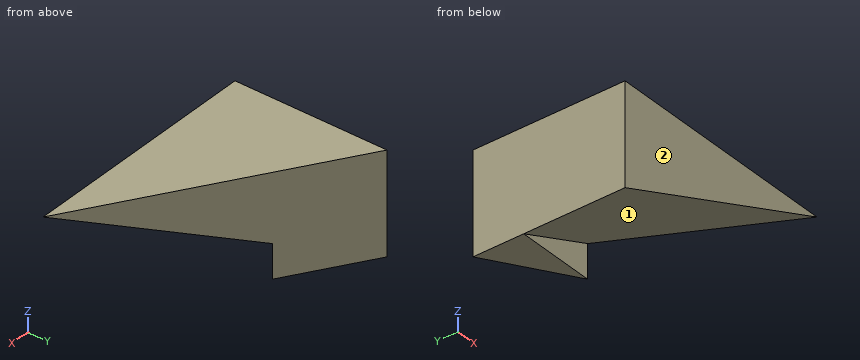
from build123d import *

# Parameters (mm, degrees)
F1_DEPTH = 25
F3_DEPTH = 25


with BuildPart() as f1:
    # F0 (on Top) → F1 (new body)
    with BuildSketch(Plane.XY):
        Polygon((-59.480719, 22.291102), (-118.588671, 59.791102), (-118.588671, 22.291102), align=None)
    extrude(amount=F1_DEPTH)

    # F2 (on face) → F3 (cut)
    with BuildSketch(Plane.XZ.offset(-22.291102)):
        Polygon((-59.480719, 25), (-118.588671, 0), (-59.480719, 0), align=None)
    extrude(amount=-F3_DEPTH, mode=Mode.SUBTRACT)


solid = f1.part
The listing builds one solid part. Answer for the finished solid, in the listing's coordinates (mm). Face numbers are marked on the shaded views. A direction names the side the tool comes from. Round coordinates to 2 decimals unless told otherwise and drop trailing zeros. Write each loop counter-clockwise with the first axis right and the second up, starting at its lowest first coordinate (ties: lowest second). Pieces come first, ordered by that corner, then holes. Notation, with made-up numbers: M -8.5,44 L 50.5,44 A17 ccw 50.5,69 Z; hole C 46.5,22 d7. An arc over 180 degrees is marked long. Write each question's results on one line, items separated by ' | '. Start each with the question number.
Item 1: Find section D-D on z = 4. Write down the section's boundary in (x, y), and give its area (3 significant figures).
Item 2: Straight lines are drawn through the part: probe 1 along X at (y, z) = (43, 1); probe 2 along Z at (x, y) = (-101.5, 41); probe 3 along Y at (x, z) = (-101, 7.25). For each, find the intervals that lie inside material, in ascending order.
Item 3: Given pin 1 Ø3 at (x, y) = (-110, 37.5) entering from -Z; pin 2 Ø4 at (x, y) = (-83, 36) entering from -Z, each flat-ended and moving along its own axis, determine where each tip first touches the part or whether it passes through.
Item 4: Find section C-C on y = 56. Write down the section's boundary in (x, z).
Item 5: Which of the six approach directions +Z, -Z, +X, -X, +Y, -Y give full straight-line access (tool end or side, diameter ignored) to the marked faces 1 and 2?
Item 6: Find section A-A on x = -104. Write down the section's boundary in (y, z), and give its area (3 significant figures).
Item 7: Find section B-B on z = 21.25. Write down the section's boundary in (x, y), and give its area (3 significant figures).
Answer block:
1) outline: M -118.59,22.29 L -109.13,22.29 L -109.13,47.29 L -98.89,47.29 L -118.59,59.79 Z | area: 360 mm²
2) probe 1: x = -118.59 to -116.22 | probe 2: z = 7.23 to 25 | probe 3: y = 47.29 to 48.63
3) pin 1: stops at z = 3 | pin 2: stops at z = 14.21
4) outline: M -118.59,0 L -112.61,0 L -112.61,25 L -118.59,25 Z
5) face 1: -Z, +X, -Y | face 2: +Z, -Z, +X, -X, -Y
6) outline: M 22.29,6.17 L 47.29,6.17 L 47.29,0 L 50.54,0 L 50.54,25 L 22.29,25 Z | area: 552 mm²
7) outline: M -118.59,22.29 L -68.35,22.29 L -68.35,27.92 L -118.59,59.79 Z | area: 1,080 mm²
